Read the model definition and answer for the solid it produces. Units are mm, in the model's axes. Face numbers are marked on the shaded views. Round coordinates to 2 decimals unless told otherwise and drop trailing zeros. Order: outer loops, then holes, each group sorted by start corner. A loop starts at its lowest first (then second) coordinate and runs counter-clockwise, first axis right, second up. Notation, with made-up numbers: (85.25, -10) -> (142.25, -10) arc R20 cw to (142.25, 7) -> close; hole circle Ø11 at (36, 23.5). An arc over 180 degrees is marked (long way). One line per item, written item: value. Start each with the question number.
1. Section B-B (y = -7) is taken. Give the vertices of the cut face in (x, z).
2. The mould has two halves that part along Y. Classify the marked faces 1, 2 and 3: released by +Y, released by -Y, zero draft, split by the parting line, or undercut.
3. Flat-ended cylindrical pins translate along their axes: pin 1 Ø1.5 at (x, y) = (-34.5, -34) entering from -Z; pin 2 Ø0.6 at (x, z) = (-37.5, -37) entering from -Y. Find the tip coordinate at first contact, or state that the pin passes through.
4. Consider line 1 (X direction, y = -26.5, z = -60); line 2 (Z direction, x = -83, y = -29.5); line 3 (X direction, y = -33, z = -64.5). Determine where each line is inside the solid, lowest interval first.
5. Section A-A (y = -29) is taken. Give the vertices of the cut face in (x, z).
from build123d import *

# Parameters (mm, degrees)
F0_W         = 127
F0_H         = 88.9
F1_DEPTH     = 38.1
F2_W         = 127
F2_H         = 38.1
F2_W_2       = 82.55
F2_H_2       = 12.954
F3_DEPTH     = 25.4
F4_DEPTH     = 25.4
F5_W         = 44.1795827687
F5_H         = 12.954
F6_DEPTH     = 81.28
F7_R         = 39.8475218447
F7_R_2       = 34.8773795478
F8_DEPTH     = 22.86
F9_T3_DEPTH  = 152.4
F9_T6_DEPTH  = 114.3
F9_T9_DEPTH  = 114.3
F9_T12_DEPTH = 152.4


# Not quite as in the source:
# - a fillet or chamfer that OpenCascade refuses, or shapes differently, is made with other operations: its cross-section is extruded or revolved along the edge and cut away or added


with BuildPart() as f1:
    # F0 (on Front) → F1 (new body)
    with BuildSketch(Plane.XZ):
        with Locations((-63.5, -31.0818182497)):
            Rectangle(F0_W, F0_H)
    extrude(amount=F1_DEPTH)

    # F2 (on face) → F3 (join)
    with BuildSketch(Plane.XY.offset(13.3681817503)):
        with Locations((-63.5, -19.05)):
            Rectangle(F2_W, F2_H)
        with Locations((-79.4304944575, -8.7889100092)):
            Rectangle(F2_W_2, F2_H_2, mode=Mode.SUBTRACT)
    extrude(amount=-F3_DEPTH)

    # F2 (on face) → F4 (cut)
    with BuildSketch(Plane.XY.offset(13.3681817503)):
        with Locations((-79.4304944575, -8.7889100092)):
            Rectangle(F2_W_2, F2_H_2)
    extrude(amount=-F4_DEPTH, mode=Mode.SUBTRACT)

    # F5 (on face) → F6 (cut)
    with BuildSketch(Plane.XY.offset(13.3681817503)):
        with Locations((-60.2452858418, -8.7889100092)):
            Rectangle(F5_W, F5_H)
    extrude(amount=-F6_DEPTH, mode=Mode.SUBTRACT)

    # F7 (on face) → F8 (cut)
    with BuildSketch(Plane.XZ.offset(38.1)):
        with Locations((-76.8643096089, -33.7820015848)):
            Circle(F7_R)
        with Locations((-76.8643096089, -33.7820015848)):
            Circle(F7_R_2, mode=Mode.SUBTRACT)
    extrude(amount=-F8_DEPTH, mode=Mode.SUBTRACT)

    # F9: fillet of radius 5.08 on 5 edges, made by hand


with BuildPart() as f9_tool1:
    # F9_s2 → F9_t3 (new body)
    with BuildSketch(Plane.YZ.offset(12.7)):
        with BuildLine():
            ThreePointArc((-38.1, 8.2881817503), (-36.6121024484, 11.8802841987), (-33.02, 13.3681817503))
            Line((-33.02, 13.3681817503), (-38.1, 13.3681817503))
            Line((-38.1, 13.3681817503), (-38.1, 8.2881817503))
        make_face()
    extrude(amount=-F9_T3_DEPTH)


with BuildPart() as f9_tool4:
    # F9_s5 → F9_t6 (new body)
    with BuildSketch(Plane.XY.offset(-88.2318182497)):
        with BuildLine():
            ThreePointArc((-5.08, -38.1), (-1.4878975516, -36.6121024484), (0, -33.02))
            Line((0, -33.02), (0, -38.1))
            Line((0, -38.1), (-5.08, -38.1))
        make_face()
    extrude(amount=F9_T6_DEPTH)


with BuildPart() as f9_tool7:
    # F9_s8 → F9_t9 (new body)
    with BuildSketch(Plane.XY.offset(26.0681817503)):
        with BuildLine():
            ThreePointArc((-121.92, -38.1), (-125.5121024484, -36.6121024484), (-127, -33.02))
            Line((-127, -33.02), (-127, -38.1))
            Line((-127, -38.1), (-121.92, -38.1))
        make_face()
    extrude(amount=-F9_T9_DEPTH)


with BuildPart() as f9_tool10:
    # F9_s11 → F9_t12 (new body)
    with BuildSketch(Plane.YZ.offset(-139.7)):
        with BuildLine():
            ThreePointArc((-38.1, -70.4518182497), (-36.6121024484, -74.0439206982), (-33.02, -75.5318182497))
            Line((-33.02, -75.5318182497), (-38.1, -75.5318182497))
            Line((-38.1, -75.5318182497), (-38.1, -70.4518182497))
        make_face()
    extrude(amount=F9_T12_DEPTH)


with BuildPart() as f9_tool13:
    # F9_s14 → F9_t15 (revolve)
    with BuildSketch(Plane.XY.offset(-33.7820015848)):
        with BuildLine():
            ThreePointArc((-31.9367877642, -38.1), (-35.5288902127, -36.6121024484), (-37.0167877642, -33.02))
            Line((-37.0167877642, -33.02), (-37.0167877642, -38.1))
            Line((-37.0167877642, -38.1), (-31.9367877642, -38.1))
        make_face()
    revolve(axis=Axis((-76.8643096089, -38.1, -33.7820015848), (0, -1, 0)))


with BuildPart() as f1_1:
    add(f1.part)

    # F9_t16: cut F9_tool1, F9_tool4, F9_tool7, F9_tool10, F9_tool13
    add([f9_tool1.part, f9_tool4.part, f9_tool7.part, f9_tool10.part, f9_tool13.part], mode=Mode.SUBTRACT)


solid = f1_1.part
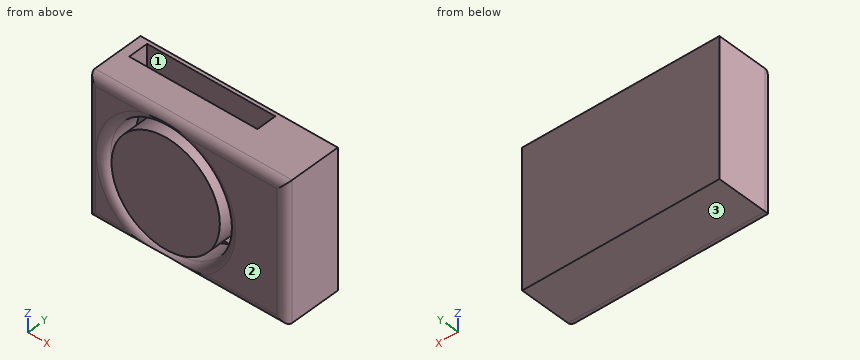
Answer:
1. outline: (-127, -75.53) -> (0, -75.53) -> (0, 13.37) -> (-38.16, 13.37) -> (-38.16, -67.91) -> (-82.34, -67.91) -> (-82.34, -12.03) -> (-120.71, -12.03) -> (-120.71, 13.37) -> (-127, 13.37) -> close
2. face 1: undercut
2. face 2: released by -Y
2. face 3: zero draft
3. pin 1: z = -75.53
3. pin 2: y = -15.24
4. line 1: -127 to -106.87, -99.87 to -53.86, -46.86 to 0
4. line 2: -75.53 to -73.15, -68.12 to 0.55, 5.59 to 13.37
4. line 3: -127 to -102.25, -93.38 to -60.35, -51.48 to 0
5. outline: (-127, -75.53) -> (0, -75.53) -> (0, 13.37) -> (-127, 13.37) -> close; circle Ø69.75 at (-76.86, -33.78); hole circle Ø79.7 at (-76.86, -33.78)
